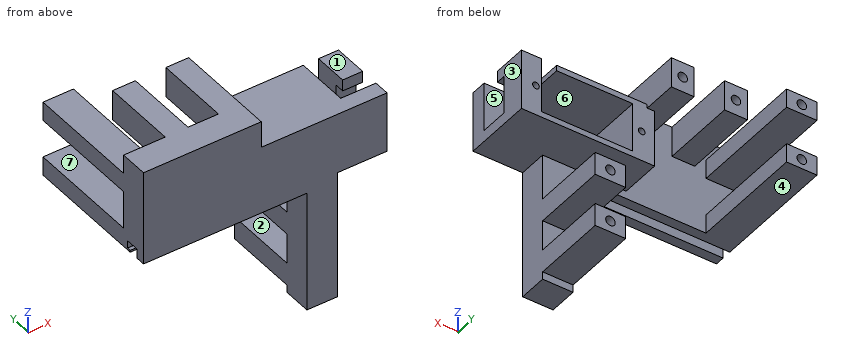
```python
from build123d import *

# Parameters (mm, degrees)
SKETCH1_W                       = 70
SKETCH1_H                       = 50
BOSS_EXTRUDE1_DEPTH             = 7.5
SKETCH2_W                       = 35
SKETCH2_H                       = 16
BOSS_EXTRUDE2_DEPTH             = 10.7
SKETCH3_W                       = 24
SKETCH3_H                       = 13
CUT_EXTRUDE1_DEPTH              = 15.7
SKETCH4_R                       = 0.875
CUT_EXTRUDE2_DEPTH              = 8
SKETCH9_W                       = 70
SKETCH9_H                       = 7.5
BOSS_EXTRUDE10_DEPTH            = 7
SKETCH10_W                      = 8
SKETCH10_H                      = 20
SKETCH10_W_2                    = 20
SKETCH10_H_2                    = 8
BOSS_EXTRUDE11_DEPTH            = 19.75
SKETCH14_W                      = 8
SKETCH14_H                      = 8
CUT_EXTRUDE4_DEPTH              = 19.75
TAP_DRILL_FOR_M3X0_5_TAP1_D     = 2.5
TAP_DRILL_FOR_M3X0_5_TAP1_DEPTH = 5
TAP_DRILL_FOR_M3X0_5_TAP1_TIP   = 0.751075774
SKETCH6_W                       = 8
SKETCH6_H                       = 20
BOSS_EXTRUDE8_DEPTH             = 30.25
SKETCH19_W                      = 8
SKETCH19_H                      = 10
CUT_EXTRUDE6_DEPTH              = 30.25
TAP_DRILL_FOR_M3X0_5_TAP3_D     = 2.5
TAP_DRILL_FOR_M3X0_5_TAP3_DEPTH = 5
TAP_DRILL_FOR_M3X0_5_TAP3_TIP   = 0.751075774
SKETCH22_W                      = 13.05
SKETCH22_H                      = 34
SKETCH22_W_2                    = 33.05
SKETCH22_H_2                    = 7
CUT_EXTRUDE7_DEPTH              = 7.5
CUT_EXTRUDE8_DEPTH              = 42.95
SKETCH25_W                      = 10
SKETCH25_H                      = 7.5
CUT_EXTRUDE9_DEPTH              = 5.25
SKETCH26_W                      = 4
SKETCH26_H                      = 14.05
CUT_EXTRUDE10_DEPTH             = 1.5
SKETCH27_W                      = 5.25
SKETCH27_H                      = 5
CUT_EXTRUDE11_DEPTH             = 3


with BuildPart() as part:
    # Sketch1 → Boss-Extrude1 (new body)
    with BuildSketch(Plane(origin=(0, 0, 0), x_dir=(1, 0, 0), z_dir=(0, 1, 0))):
        Rectangle(SKETCH1_W, SKETCH1_H)
    extrude(amount=BOSS_EXTRUDE1_DEPTH)

    # Sketch2 → Boss-Extrude2 (add)
    with BuildSketch(Plane(origin=(0, 7.5, 0), x_dir=(1, 0, 0), z_dir=(0, 1, 0))):
        with Locations((17.5, -17)):
            Rectangle(SKETCH2_W, SKETCH2_H)
    extrude(amount=BOSS_EXTRUDE2_DEPTH)

    # Sketch3 → Cut-Extrude1 (cut)
    with BuildSketch(Plane(origin=(0, 18.2, 0), x_dir=(1, 0, 0), z_dir=(0, 1, 0))):
        with Locations((17.75, -17)):
            Rectangle(SKETCH3_W, SKETCH3_H)
    extrude(amount=-CUT_EXTRUDE1_DEPTH, mode=Mode.SUBTRACT)

    # Sketch4 → Cut-Extrude2 (cut)
    with BuildSketch(Plane(origin=(0, 18.2, 0), x_dir=(1, 0, 0), z_dir=(0, 1, 0))):
        with Locations(Location((3.4, -17, 0), (0, 0, 270))):
            Circle(SKETCH4_R)
        with Locations(Location((31.2, -17, 0), (0, 0, 270))):
            Circle(SKETCH4_R)
    extrude(amount=-CUT_EXTRUDE2_DEPTH, mode=Mode.SUBTRACT)

    # Sketch9 → Boss-Extrude10 (add)
    with BuildSketch(Plane.XY.offset(25)):
        with Locations((0, 3.75)):
            Rectangle(SKETCH9_W, SKETCH9_H)
    extrude(amount=BOSS_EXTRUDE10_DEPTH)

    # Sketch10 → Boss-Extrude11 (add)
    with BuildSketch(Plane(origin=(0, 7.5, 0), x_dir=(1, 0, 0), z_dir=(0, 1, 0))):
        with Locations((17.95, 13)):
            Rectangle(SKETCH10_W, SKETCH10_H)
        with Locations((-8.05, -28)):
            Rectangle(SKETCH10_W_2, SKETCH10_H_2)
    extrude(amount=BOSS_EXTRUDE11_DEPTH)

    # Sketch14 → Cut-Extrude4 (cut)
    with BuildSketch(Plane(origin=(0, 27.25, 0), x_dir=(1, 0, 0), z_dir=(0, 1, 0))):
        with Locations((-8.05, -28)):
            Rectangle(SKETCH14_W, SKETCH14_H)
        with Locations((17.95, 13)):
            Rectangle(SKETCH14_W, SKETCH14_H)
    extrude(amount=-CUT_EXTRUDE4_DEPTH, mode=Mode.SUBTRACT)

    # Tap Drill for M3x0.5 Tap1
    with Locations(Plane(origin=(-15.05, 27.25, 28), x_dir=(0, 0, 1), z_dir=(0, 1, 0))):
        with Locations((0, 0), (0, 14), (-34, 33), (-48, 33)):
            Hole(TAP_DRILL_FOR_M3X0_5_TAP1_D / 2, depth=TAP_DRILL_FOR_M3X0_5_TAP1_DEPTH)
            with Locations((0, 0, -(TAP_DRILL_FOR_M3X0_5_TAP1_DEPTH + TAP_DRILL_FOR_M3X0_5_TAP1_TIP / 2))):  # 118° drill point
                Cone(0, TAP_DRILL_FOR_M3X0_5_TAP1_D / 2, TAP_DRILL_FOR_M3X0_5_TAP1_TIP, mode=Mode.SUBTRACT)

    # Sketch6 → Boss-Extrude8 (add)
    with BuildSketch(Plane(origin=(0, 7.5, 0), x_dir=(1, 0, 0), z_dir=(0, 1, 0))):
        with Locations((-25, -17)):
            Rectangle(SKETCH6_W, SKETCH6_H)
    extrude(amount=BOSS_EXTRUDE8_DEPTH)

    # Sketch19 → Cut-Extrude6 (cut)
    with BuildSketch(Plane(origin=(0, 37.75, 0), x_dir=(1, 0, 0), z_dir=(0, 1, 0))):
        with Locations((-25, -17)):
            Rectangle(SKETCH19_W, SKETCH19_H)
    extrude(amount=-CUT_EXTRUDE6_DEPTH, mode=Mode.SUBTRACT)

    # Tap Drill for M3x0.5 Tap3
    with Locations(Plane(origin=(-25, 37.75, 9.5), x_dir=(0, 0, 1), z_dir=(0, 1, 0))):
        with Locations((0, 0), (15, 0)):
            Hole(TAP_DRILL_FOR_M3X0_5_TAP3_D / 2, depth=TAP_DRILL_FOR_M3X0_5_TAP3_DEPTH)
            with Locations((0, 0, -(TAP_DRILL_FOR_M3X0_5_TAP3_DEPTH + TAP_DRILL_FOR_M3X0_5_TAP3_TIP / 2))):  # 118° drill point
                Cone(0, TAP_DRILL_FOR_M3X0_5_TAP3_D / 2, TAP_DRILL_FOR_M3X0_5_TAP3_TIP, mode=Mode.SUBTRACT)

    # Sketch22 → Cut-Extrude7 (cut)
    with BuildSketch(Plane(origin=(0, 7.5, 0), x_dir=(1, 0, 0), z_dir=(0, 1, 0))):
        Polygon((13.95, -7), (13.95, 25), (-35, 25), (-35, -32), (-29, -32), (-29, -7), align=None)
        with Locations((28.475, 8)):
            Rectangle(SKETCH22_W, SKETCH22_H)
        with Locations((18.475, -28.5)):
            Rectangle(SKETCH22_W_2, SKETCH22_H_2)
    extrude(amount=-CUT_EXTRUDE7_DEPTH, mode=Mode.SUBTRACT)

    # Sketch24 → Cut-Extrude8 (cut)
    with BuildSketch(Plane.ZY.offset(29)):
        Polygon((7, 2.5), (9.5, 2.5), (9.5, 6), (7.5, 6), (7.5, 5), (7, 5), align=None)
    extrude(amount=-CUT_EXTRUDE8_DEPTH, mode=Mode.SUBTRACT)

    # Sketch25 → Cut-Extrude9 (cut)
    with BuildSketch(Plane.ZY.offset(-29.75)):
        with Locations((17, 7.9)):
            Rectangle(SKETCH25_W, SKETCH25_H)
    extrude(amount=-CUT_EXTRUDE9_DEPTH, mode=Mode.SUBTRACT)

    # Sketch26 → Cut-Extrude10 (cut)
    with BuildSketch(Plane.XY.offset(25)):
        with Locations((27.75, 11.175)):
            Rectangle(SKETCH26_W, SKETCH26_H)
    extrude(amount=-CUT_EXTRUDE10_DEPTH, mode=Mode.SUBTRACT)

    # Sketch27 → Cut-Extrude11 (cut)
    with BuildSketch(Plane.XY.offset(25)):
        with Locations((32.375, 6.65)):
            Rectangle(SKETCH27_W, SKETCH27_H)
    extrude(amount=-CUT_EXTRUDE11_DEPTH, mode=Mode.SUBTRACT)


solid = part.part
```
Geometry: final body of the model. Coordinates: model frame, mm. Face numbers are marked on the shaded views. A direction names the side the tool comes from. Coordinates: 2 decimals unless noted, no trailing zeros. Order: outer loops, then holes, each group sorted by start corner. A loop starts at its lowest first (then second) coordinate and runs counter-clockwise, first axis right, second up. Notation, with made-up numbers: (21, 49) -> (60, 49) arc R37 cw to (60, 86) -> close; hole circle Ø6 at (11, 65). An arc over 180 degrees is marked (long way). Write item = value, one per line.
(1) Cut plane C-C on y = 33.5. Return loops of the section in (x, z), plus the area to 3 significant figures.
Solved:
outline = (-29, 7) -> (-21, 7) -> (-21, 12) -> (-29, 12) -> close; (-29, 22) -> (-21, 22) -> (-21, 27) -> (-29, 27) -> close; hole circle Ø2.5 at (-25, 9.5); hole circle Ø2.5 at (-25, 24.5)
area = 70.2 mm²
(2) Pull-direction query (Z, two-part tool) for the marked faces 1, 2, 3 and 4; classes: pulls with the +Z half, pulls with the -Z half, needs draft (parallel to the pull), parting line crosses it, or undercut.
Solved:
face_1 = pulls with the +Z half
face_2 = undercut
face_3 = needs draft
face_4 = pulls with the -Z half
(3) Pin query (flat end, axial travel): pin 1 Ø6 at (y, z) = (26.5, -2.5) entering from +X; pin 2 Ø10 at (x, y) = (-11, 26.5) entering from -Z; pin 3 Ø9 at (y, z) = (21.5, 28.5) entering from +X; pin 4 Ø6 at (x, y) = (6.5, 30) entering from -Z. Return the tip coordinate at first contact, or that it passes through.
Solved:
pin_1 = 21.95
pin_2 = 24
pin_3 = 1.95
pin_4 = through
(4) Access query for the marked faces 5, 6 and 7. Directions: +Z, -Z, +X, -X, +Y, -Y. A direction counts if a zero-diameter tool reaches every point of the face in a straight line with its end or side. Return the directions, or none.
Solved:
face_5 = +Z, +X
face_6 = +Y
face_7 = -X, +Y
(5) Cut plane A-A on y = 19. Return loops of the section in (x, z).
Solved:
outline = (-29, 7) -> (-21, 7) -> (-21, 12) -> (-29, 12) -> close; (-29, 22) -> (-21, 22) -> (-21, 27) -> (-29, 27) -> close; (-18.05, 24) -> (-12.05, 24) -> (-12.05, 32) -> (-18.05, 32) -> close; (-4.05, 24) -> (1.95, 24) -> (1.95, 32) -> (-4.05, 32) -> close; (13.95, -23) -> (21.95, -23) -> (21.95, -17) -> (13.95, -17) -> close; (13.95, -9) -> (21.95, -9) -> (21.95, -3) -> (13.95, -3) -> close
(6) Cut plane B-B on x = 31.2. Return loops of the section in (y, z) (3 decimals).
Solved:
outline = (0, 9) -> (18.2, 9) -> (18.2, 16.125) -> (11.65, 16.125) -> (11.65, 12) -> (4.15, 12) -> (4.15, 25) -> (0, 25) -> close; (9.15, 22) -> (11.65, 22) -> (11.65, 17.875) -> (18.2, 17.875) -> (18.2, 25) -> (9.15, 25) -> close
(7) Line query: line 1 (X direction, y = 25.9, z = 28); line 2 (Z direction, x = 17.95, y = 24.2); line 3 (Z direction, x = -25, y = 34). Output: solid intervals per line, ascending.
Solved:
line_1 = -18.05 to -16.3, -13.8 to -12.05, -4.05 to -2.3, 0.2 to 1.95
line_2 = -23 to -21.25, -18.75 to -17, -9 to -7.25, -4.75 to -3
line_3 = 7 to 8.25, 10.75 to 12, 22 to 23.25, 25.75 to 27
(8) Cut plane D-D on x = 12.5. Return loops of the section in (y, z).
Solved:
outline = (0, 7) -> (2.5, 7) -> (2.5, 9.5) -> (6, 9.5) -> (6, 7.5) -> (5, 7.5) -> (5, 7) -> (7.5, 7) -> (7.5, 9) -> (18.2, 9) -> (18.2, 10.5) -> (2.5, 10.5) -> (2.5, 23.5) -> (18.2, 23.5) -> (18.2, 25) -> (0, 25) -> close
